The figure shows three views and two pictorial views of one solid part (mm, origin at its lowest corner). Answer the questions. A direction names the side the tool comes from. Round coordinates to 2 decimals unless told otherwise and drop trailing zeros. Loops run counter-clockwise (first coordinate to the right, second up) from the corner with the lowest first, then second, coordinate; pieces in that order, holes last. Notation, with made-up numbers: (80, -2.5) -> (88, -2.5) arc R10 cw to (88, 6.5) -> close; hole circle Ø1 at (5.25, 26). An arc over 180 degrees is marked (long way). Use a Markdown table: item, result. Add a question column.
Q1. Which of the six approach directions +Z, -Z, +X, -X, +Y, -Y give full straight-line access (tool end or side, diameter ignored) to the marked faces 4 and 5?
Q2. Given pin 1 Ø1.5 at (y, z) = (9.5, 1) entering from +X, flat-ended and moving along its own axis, determine where the tip first touches the part or whether it passes through.
Q3. Section C-C on z = 3.85 is taken. Give the vertices of the cut face in (x, y).
Q4. Section D-D on z = 1.35 is taken. Give the vertices of the cut face in (x, y).
Q5. Section A-A on y = 5.5 is taken. Give the vertices of the cut face in (x, z).
Q6. For a pull along X with two mould halves and no side action, classify the marked faces 1, 2 and 3 as released by +X, released by -X, zero draft, split by the parting line, or undercut.
Q7. Consider line 1 (Y direction, x = 5.5, z = 2.15); line 2 (Z direction, x = 8.75, y = 2.25); line 3 (X direction, y = 6.75, z = 4.85) (1 decimal). Determine where each line is inside the solid, lowest interval first.
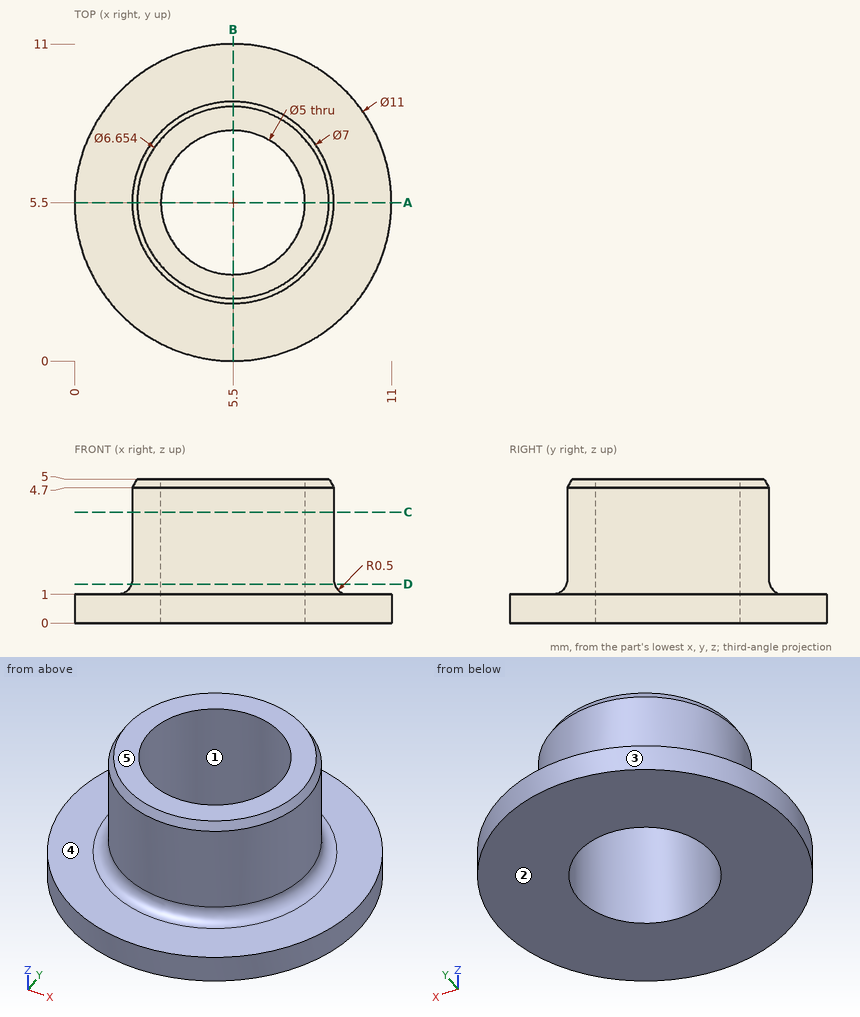
Checked values:
| question | item | result |
|---|---|---|
| 1 | face 4 | +Z |
| 1 | face 5 | +Z, +X, -X, +Y, -Y |
| 2 | pin 1 | stops at x = 9.94 |
| 3 | outline | circle Ø7 at (5.5, 5.5); hole circle Ø5 at (5.5, 5.5) |
| 4 | outline | circle Ø7.05 at (5.5, 5.5); hole circle Ø5 at (5.5, 5.5) |
| 5 | outline | (0, 0) -> (3, 0) -> (3, 5) -> (2.17, 5) -> (2, 4.7) -> (2, 1.5) arc R0.5 cw to (1.5, 1) -> (0, 1) -> close; (8, 0) -> (11, 0) -> (11, 1) -> (9.5, 1) arc R0.5 cw to (9, 1.5) -> (9, 4.7) -> (8.83, 5) -> (8, 5) -> close |
| 6 | face 1 | undercut |
| 6 | face 2 | zero draft |
| 6 | face 3 | split by the parting line |
| 7 | line 1 | y = 2 to 3, 8 to 9 |
| 7 | line 2 | z = 0 to 1 |
| 7 | line 3 | x = 2.3 to 3.3, 7.7 to 8.7 |
